For this review, take the finished solid that the model builds, in its own axes (mm). A direction names the side the tool comes from. Round coordinates to 2 decimals unless told otherwise and drop trailing zeros. Order: outer loops, then holes, each group sorted by start corner. A loop starts at its lowest first (then second) coordinate and runs counter-clockwise, first axis right, second up. Notation, with made-up numbers: M -29.75,29 L 1.25,29 A11 ccw 1.25,48 Z; hole C 41,64 d7. An arc over 180 degrees is marked long. Answer as a JSON object with one key per item and string values.
from build123d import *

# Parameters (mm, degrees)
F0_W          = 170.18
F0_H          = 132.08
F0_W_2        = 132.08
F0_H_2        = 93.98
F1_DEPTH      = 9.525
F2_W          = 19.05
F2_H          = 19.05
F3_DEPTH      = 101.6
F3_DEPTH_BACK = 127


with BuildPart() as f1:
    # F0 (on Top) → F1 (new body, symmetric)
    with BuildSketch(Plane.XY):
        Rectangle(F0_W, F0_H)
        Rectangle(F0_W_2, F0_H_2, mode=Mode.SUBTRACT)
    extrude(amount=F1_DEPTH, both=True)

    # F2 (on face) → F3 (join, two sides)
    with BuildSketch(Plane(origin=(0, 0, -9.525), x_dir=(1, 0, 0), z_dir=(0, 0, -1))) as f3_sk:
        with Locations((0, -56.515)):
            Rectangle(F2_W, F2_H)
    extrude(amount=F3_DEPTH)
    extrude(f3_sk.sketch, amount=-F3_DEPTH_BACK)


solid = f1.part
1) Add section C-C on z = 70. State the section outline as (x, y) points (3 decimals), and give its area (3 significant figures).
Geometry check:
{"outline": "M -9.525,46.99 L 9.525,46.99 L 9.525,66.04 L -9.525,66.04 Z", "area": "363 mm²"}
2) Add section A-A on y = -28. State the section outline as (x, z) points (3 decimals), and give its area (3 significant figures).
Geometry check:
{"outline": "M -85.09,-9.525 L -66.04,-9.525 L -66.04,9.525 L -85.09,9.525 Z; M 66.04,-9.525 L 85.09,-9.525 L 85.09,9.525 L 66.04,9.525 Z", "area": "726 mm²"}
3) Mouldability with a two-part tool opening along X and no side actions: class faces 4 (the flat face through (5, 46.99, 4)), 5 (the flat face through (85.09, -1, 0)), 6 (the flat face through (-1, -58, 9.525)) as +X half, -X half, draft (parallel to the pull), parting line (faces both ways), or undercut.
Geometry check:
{"face 4": "undercut", "face 5": "+X half", "face 6": "draft"}
4) For L1, parallel to X at y = -28.5, z = -9; L2, parallel to Z at x = 67, y = -8 (3 decimals); L3, parallel to Y at x = 5, z = 75.5, list the stretches that pass through material, from the lowest coordinate up.
Geometry check:
{"L1": "x = -85.09 to -66.04, 66.04 to 85.09", "L2": "z = -9.525 to 9.525", "L3": "y = 46.99 to 66.04"}
5) Machinability: for faces 1 (the flat face through (-66.04, -1, 0)), 2 (the flat face through (-9.525, 57, -60)), 3 (the flat face through (9.525, 57, 63)), which of the approach directions +Z, -Z, +X, -X, +Y, -Y give a long, thin tool a straight path to every point of the face, cutting with its end or side? Answer none if there is none.
Geometry check:
{"face 1": "+Z, -Z", "face 2": "-Z, -X, +Y, -Y", "face 3": "+Z, +X, +Y, -Y"}
6) Add section D-D on y = -57.5. State the section outline as (x, z) points (3 decimals).
Geometry check:
{"outline": "M -85.09,-9.525 L 85.09,-9.525 L 85.09,9.525 L -85.09,9.525 Z"}
7) Insertion check: P1, Ø9.5, axis at y = 53, z = 61.5, coming from the -X side (3 decimals); P2, Ø15, axis at y = 61, z = -55.5, coming from the +X side (3 decimals); P3, Ø4, axis at x = 59.5, y = 44.5, coming from the +Z side. Each pin has a flat end and moves straight along its axis. Give the tip position at first contact, or say it passes through.
Geometry check:
{"P1": "stops at x = -9.525", "P2": "stops at x = 9.525", "P3": "passes through"}
8) Add section B-B on x = 22. State the section outline as (y, z) points (3 decimals).
Geometry check:
{"outline": "M -66.04,-9.525 L -46.99,-9.525 L -46.99,9.525 L -66.04,9.525 Z; M 46.99,-9.525 L 66.04,-9.525 L 66.04,9.525 L 46.99,9.525 Z"}
